Input: part model. Units: mm. Frame: model coordinates. Face numbers are marked on the shaded views. A direction names the side the tool comes from. Coordinates: 2 decimals unless noted, no trailing zeros. Write each loop counter-clockwise with the first axis right and the second up, starting at its lowest first coordinate (ties: lowest second). Pieces come first, ordered by that corner, then holes. Notation, with made-up numbers: (1, -10) -> (41, -10) arc R23 cw to (41, -1) -> close; hole circle Ø9 at (15.5, 62.25). An arc over 180 degrees is marked (long way). Use one line per item in the form item = value. Start each with the question number.
(1) Cut plane D-D on z = -9.5. Return the cut outline in (x, y) (3 decimals), plus the area to 3 significant figures.
(2) Set-up query: the marked faces 1, 2 and 3. Return all of +Z, -Z, +X, -X, +Y, -Y with unobstructed straight access to the full face (end or side cutting, diameter ignored); none if empty.
(3) Cut plane A-A on z = -4.75. Return the cut outline in (x, y), plus the area to 3 significant figures.
(4) First-contact query: pin 1 (7 mm diameter, centred on y = -26.5, z = -3, fed in from -X); pin 2 (1.4 mm diameter, centred on y = -30, z = -19.5, fed in from +X); pin 3 (2 mm diameter, centred on y = -17.5, z = -5, fed in from +X); pin 4 (4 mm diameter, centred on x = 36, z = -5, fed in from -Y). Flat tips, straight axial feed; report the tip coordinate or a pass-through.
(5) Cut plane C-C on y = -18.5. Return the cut outline in (x, z).
(6) Ray query, line 1 along X through (y, z) = (-29.5, -14.25); line 2 along Y through (x, z) = (53.5, -19.25); line 3 along X through (y, z) = (-13.5, -9.75). Return the intervals inside material, ascending.
(7) Cut plane B-B on x = 18. Return the cut outline in (y, z).
```python
from build123d import *

# Parameters (mm, degrees)
SKETCH1_W           = 21.59
SKETCH1_H           = 36.83
BOSS_EXTRUDE1_DEPTH = 127
SKETCH2_W           = 50.8
SKETCH2_H           = 25.4
CUT_EXTRUDE1_DEPTH  = 25.4
SKETCH3_W           = 63.5
SKETCH3_H           = 22.86
CUT_EXTRUDE2_DEPTH  = 22.86
SKETCH4_W           = 6.35
SKETCH4_H           = 8.382
CUT_EXTRUDE3_DEPTH  = 69.85
SKETCH5_W           = 6.35
SKETCH5_H           = 8.89
CUT_EXTRUDE4_DEPTH  = 69.85
SKETCH6_W           = 6.096
SKETCH6_H           = 13.97
CUT_EXTRUDE5_DEPTH  = 13.208
SKETCH7_W           = 6.205413724
SKETCH7_H           = 13.97
CUT_EXTRUDE6_DEPTH  = 13.208
SKETCH8_R           = 3.302
CUT_EXTRUDE7_DEPTH  = 13.208
FILLET1_R           = 6.35
FILLET2_R           = 6.35
FILLET3_R           = 6.35
FILLET4_R           = 6.35
FILLET5_R           = 6.35
FILLET6_R           = 6.35
SKETCH9_W           = 15.24
SKETCH9_H           = 8.89
BOSS_EXTRUDE2_DEPTH = 25.4


with BuildPart() as part:
    # Sketch1 → Boss-Extrude1 (new body)
    with BuildSketch(Plane(origin=(0, 0, 0), x_dir=(0, 0, -1), z_dir=(1, 0, 0))):
        with Locations((10.795, -18.415)):
            Rectangle(SKETCH1_W, SKETCH1_H)
    extrude(amount=BOSS_EXTRUDE1_DEPTH)

    # Sketch2 → Cut-Extrude1 (cut)
    with BuildSketch(Plane.XY):
        with Locations((25.4, -24.13)):
            Rectangle(SKETCH2_W, SKETCH2_H)
    extrude(amount=-CUT_EXTRUDE1_DEPTH, mode=Mode.SUBTRACT)

    # Sketch3 → Cut-Extrude2 (cut)
    with BuildSketch(Plane.XY):
        with Locations((95.25, -11.43)):
            Rectangle(SKETCH3_W, SKETCH3_H)
    extrude(amount=-CUT_EXTRUDE2_DEPTH, mode=Mode.SUBTRACT)

    # Sketch4 → Cut-Extrude3 (cut)
    with BuildSketch(Plane.ZY):
        with Locations((-18.415, -7.239)):
            Rectangle(SKETCH4_W, SKETCH4_H)
    extrude(amount=-CUT_EXTRUDE3_DEPTH, mode=Mode.SUBTRACT)

    # Sketch5 → Cut-Extrude4 (cut)
    with BuildSketch(Plane.ZY):
        with Locations((-3.175, -6.985)):
            Rectangle(SKETCH5_W, SKETCH5_H)
    extrude(amount=-CUT_EXTRUDE4_DEPTH, mode=Mode.SUBTRACT)

    # Sketch6 → Cut-Extrude5 (cut)
    with BuildSketch(Plane(origin=(127, 0, 0), x_dir=(0, 0, -1), z_dir=(1, 0, 0))):
        with Locations((3.048, -29.845)):
            Rectangle(SKETCH6_W, SKETCH6_H)
    extrude(amount=-CUT_EXTRUDE5_DEPTH, mode=Mode.SUBTRACT)

    # Sketch7 → Cut-Extrude6 (cut)
    with BuildSketch(Plane(origin=(127, 0, 0), x_dir=(0, 0, -1), z_dir=(1, 0, 0))):
        with Locations((18.487293138, -29.845)):
            Rectangle(SKETCH7_W, SKETCH7_H)
    extrude(amount=-CUT_EXTRUDE6_DEPTH, mode=Mode.SUBTRACT)

    # Sketch8 → Cut-Extrude7 (cut)
    with BuildSketch(Plane.XY.offset(-6.096)):
        with Locations((120.396, -29.845)):
            Circle(SKETCH8_R)
    extrude(amount=-CUT_EXTRUDE7_DEPTH, mode=Mode.SUBTRACT)

    # Fillet1
    fillet1_edges = [part.edges().sort_by_distance(p)[0] for p in [
        (113.792, -22.86, -3.048),
    ]]
    fillet(fillet1_edges, radius=FILLET1_R)

    # Fillet2
    fillet2_edges = [part.edges().sort_by_distance(p)[0] for p in [
        (113.792, -36.83, -3.048),
    ]]
    fillet(fillet2_edges, radius=FILLET2_R)

    # Fillet3
    fillet3_edges = [part.edges().sort_by_distance(p)[0] for p in [
        (113.792, -22.86, -18.487293138),
    ]]
    fillet(fillet3_edges, radius=FILLET3_R)

    # Fillet4
    fillet4_edges = [part.edges().sort_by_distance(p)[0] for p in [
        (113.792, -36.83, -18.487293138),
    ]]
    fillet(fillet4_edges, radius=FILLET4_R)

    # Fillet5
    fillet5_edges = [part.edges().sort_by_distance(p)[0] for p in [
        (127, -22.86, -10.740293138),
    ]]
    fillet(fillet5_edges, radius=FILLET5_R)

    # Fillet6
    fillet6_edges = [part.edges().sort_by_distance(p)[0] for p in [
        (127, -36.83, -10.740293138),
    ]]
    fillet(fillet6_edges, radius=FILLET6_R)

    # Sketch9 → Boss-Extrude2 (add)
    with BuildSketch(Plane.XZ.offset(11.43)):
        with Locations((43.18, -10.795)):
            Rectangle(SKETCH9_W, SKETCH9_H)
    extrude(amount=BOSS_EXTRUDE2_DEPTH)


solid = part.part
```
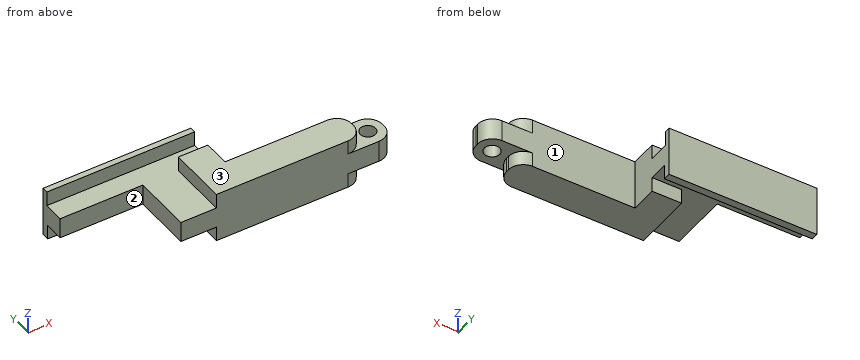
Values:
q1.outline = (0, -11.43) -> (35.56, -11.43) -> (35.56, -36.83) -> (120.65, -36.83) arc R6.35 ccw to (127, -30.48) -> (127, -29.21) arc R6.35 ccw to (120.65, -22.86) -> (63.5, -22.86) -> (63.5, 0) -> (0, 0) -> close; hole circle Ø6.604 at (120.396, -29.845)
q1.area = 2,270 mm2
q2.face_1 = +Z, -Z, +X, +Y
q2.face_2 = +Z, -Z, -X, -Y
q2.face_3 = +Z, +X, -X, +Y, -Y
q3.outline = (0, -2.54) -> (63.5, -2.54) -> (63.5, 0) -> (0, 0) -> close; (50.8, -36.83) -> (107.44, -36.83) arc R6.35 ccw to (113.79, -30.48) -> (113.79, -29.21) arc R6.35 ccw to (107.44, -22.86) -> (63.5, -22.86) -> (63.5, -11.43) -> (50.8, -11.43) -> close
q3.area = 1,170 mm2
q4.pin_1 = 35.56
q4.pin_2 = 113.79
q4.pin_3 = 63.5
q4.pin_4 = -36.83
q5.outline = (35.56, -15.24) -> (50.8, -15.24) -> (50.8, -21.59) -> (63.5, -21.59) -> (63.5, 0) -> (50.8, 0) -> (50.8, -6.35) -> (35.56, -6.35) -> close
q6.line_1 = 35.56 to 117.11, 123.68 to 127
q6.line_2 = -36.83 to -11.43, -3.05 to 0
q6.line_3 = 35.56 to 63.5
q7.outline = (-11.43, -15.24) -> (-3.05, -15.24) -> (-3.05, -21.59) -> (0, -21.59) -> (0, 0) -> (-2.54, 0) -> (-2.54, -6.35) -> (-11.43, -6.35) -> close
